```python
from build123d import *

# Parameters (mm, degrees)
F0_R     = 5.08
F0_R_2   = 1.651
F1_DEPTH = 6.35
F2_R     = 1.5875
F3_R     = 3.4925
F3_R_2   = 1.651
F4_DEPTH = 1.5875


with BuildPart() as f1:
    # F0 (on Right) → F1 (new body)
    with BuildSketch(Plane.YZ):
        Circle(F0_R)
        Circle(F0_R_2, mode=Mode.SUBTRACT)
    extrude(amount=F1_DEPTH)

    # F2
    f2_edges = [f1.edges().sort_by_distance(p)[0] for p in [
        (6.35, -5.08, 0),
        (0, -5.08, 0),
    ]]
    fillet(f2_edges, radius=F2_R)

    # F3 (on face) → F4 (cut)
    with BuildSketch(Plane.YZ.offset(6.35)):
        Circle(F3_R)
        Circle(F3_R_2, mode=Mode.SUBTRACT)
    extrude(amount=-F4_DEPTH, mode=Mode.SUBTRACT)


solid = f1.part
```
The listing builds one solid part. Answer for the finished solid, in the listing's coordinates (mm). A direction names the side the tool comes from. Round coordinates to 2 decimals unless told otherwise and drop trailing zeros. Order: outer loops, then holes, each group sorted by start corner. A loop starts at its lowest first (then second) coordinate and runs counter-clockwise, first axis right, second up. Notation, with made-up numbers: (2.5, -30) - (41.5, -30) arc R17 ccw to (41.5, -11) - close; hole circle Ø8 at (9, 81.5). An arc over 180 degrees is marked (long way). Put each result on its own line as item: value. Start each with the question number.
(1) Given P1, Ø4, axis at y = 0, z = 0.5, coming from the +X side; P2, Ø2, axis at x = 3, z = 2, coming from the -Y side; P3, Ø1.5, axis at x = 1.5, y = -3, coming from the +Z side, each flat-ended and moving along its own axis, determine where each tip first touches the part or whether it passes through.
(2) Find section D-D (x = 0.5). Give the vertices of the cut face in (y, z), plus the area to 3 significant figures.
(3) Straight lines are drawn through the part: probe 1 along Z at (x, y) = (2.15, 0); probe 2 along Z at (x, y) = (5.9, 0); probe 3 along Y at (x, z) = (2.5, -0.5). For each, find the intervals that lie inside material, in ascending order. Write a range as from..to.
(4) Determine the mould class of faces 1 (the flat face through (4.762, 2, -1)), 2 (the cylindrical face through (3.153, -0.661, 5.037)), 3 (the flat face through (0, 2, -1)) for opening direction Z: released by +Z, released by -Z, zero draft, split by the parting line, or undercut.
(5) For faces 4 (the cylindrical face through (5.567, -0.455, 3.463)), 5 (the cylindrical face through (2.348, 1.525, -0.632)), determine the directions among +Z, -Z, +X, -X, +Y, -Y from which every point of the face is accessible in a straight line to the end or side of a thin tool.
(6) Find section C-C (x = 4.5). Give the vertices of the cut face in (y, z).
Reply:
1. P1: x = 4.76
1. P2: y = -4.98
1. P3: z = 4.55
2. outline: circle Ø9.3 at (0, 0); hole circle Ø3.3 at (0, 0)
2. area: 59.3 mm^2
3. probe 1: -5.08..-1.65, 1.65..5.08
3. probe 2: -4.6..-3.49, 3.49..4.6
3. probe 3: -5.06..-1.57, 1.57..5.06
4. face 1: undercut
4. face 2: split by the parting line
4. face 3: zero draft
5. face 4: +X
5. face 5: +X, -X
6. outline: circle Ø10.16 at (0, 0); hole circle Ø3.3 at (0, 0)
